For this review, use the dimensioned drawing (mm, ordinates from the lowest corner) and the shaded views. A direction names the side the tool comes from. Coordinates: 2 decimals unless noted, no trailing zeros. Write each loop counter-clockwise with the first axis right and the second up, starting at its lowest first coordinate (ties: lowest second). Pieces come first, ordered by that corner, then holes. Notation, with made-up numbers: M 4.5,26.5 L 54.5,26.5 A13 ccw 54.5,34.5 Z; hole C 88.25,-25.5 d7. An arc over 180 degrees is marked long. Return JSON: item names as keys, results as strings.
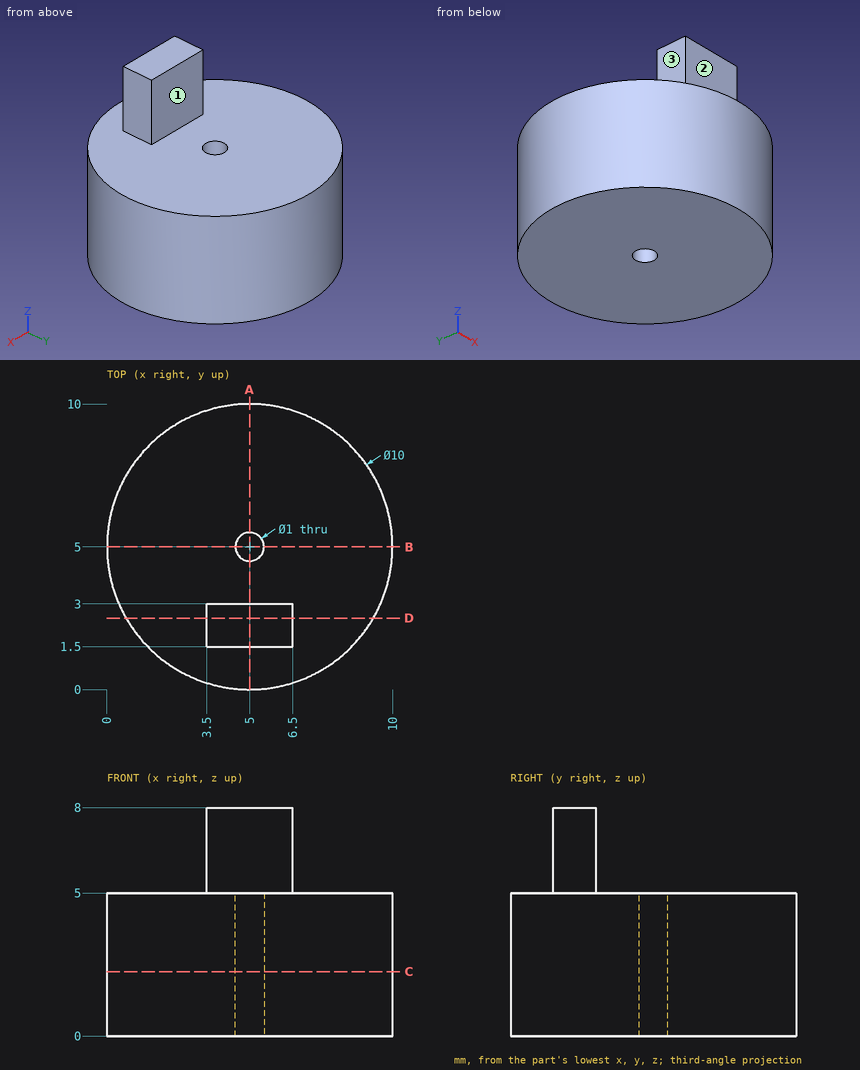
1. We need section D-D (y = 2.5). State the section outline as (x, z) points.
Checks:
{"outline": "M 0.67,0 L 9.33,0 L 9.33,5 L 6.5,5 L 6.5,8 L 3.5,8 L 3.5,5 L 0.67,5 Z"}
2. Clearance check with flat-ended pins moving along their axes: pin 1 Ø1.2 at (y, z) = (2, 6) entering from +X; pin 2 Ø1.5 at (x, z) = (5.5, 6.5) entering from -Y; pin 3 Ø0.9 at (x, z) = (5.5, 6) entering from +Y. State where each tip first meets the part, or that it passes through.
Checks:
{"pin 1": "x = 6.5", "pin 2": "y = 1.5", "pin 3": "y = 3"}
3. Wall thickness on L1, parallel to Y at x = 5, z = 2.9; L2, parallel to Z at x = 3.75, y = 1; L3, parallel to Y at x = 5.75, z = 6: over which ranges is each line inside the solid? List them lowest first. Write a range as from..to.
Checks:
{"L1": "0..4.5, 5.5..10", "L2": "0..5", "L3": "1.5..3"}
4. We need section B-B (y = 5). State the section outline as (x, z) points.
Checks:
{"outline": "M 0,0 L 4.5,0 L 4.5,5 L 0,5 Z; M 5.5,0 L 10,0 L 10,5 L 5.5,5 Z"}
5. For the marked faces 1, 2 and 3, list the 3-axis set-ups (+Z, -Z, +X, -X, +Y, -Y) from which the entire face can be reached by the end or side of a thin tool; tool diameter is ignored.
Checks:
{"face 1": "+Z, +X, -X, +Y", "face 2": "+Z, +X, -X, -Y", "face 3": "+Z, -X, +Y, -Y"}
6. We need section A-A (x = 5). State the section outline as (y, z) points, plus the area to 3 significant figures.
Checks:
{"outline": "M 0,0 L 4.5,0 L 4.5,5 L 3,5 L 3,8 L 1.5,8 L 1.5,5 L 0,5 Z; M 5.5,0 L 10,0 L 10,5 L 5.5,5 Z", "area": "49.5 mm2"}
7. We need section C-C (z = 2.25). State the section outline as (x, y) points, plus the area to 3 significant figures.
Checks:
{"outline": "C 5,5 d10; hole C 5,5 d1", "area": "77.8 mm2"}
